from build123d import *

# Parameters (mm, degrees)
SKETCH002_R            = 1.6
PAD_DEPTH              = 2
CHAMFER_SIZE           = 1.65
CHAMFER003_SIZE        = 1.65
SKETCH005_W            = 15.232
SKETCH005_H            = 21.56
SKETCH005_W_2          = 2.5
SKETCH005_H_2          = 2.6
PAD003_DEPTH           = 2
SKETCH_R               = 3.8
SKETCH_R_2             = 1.6
PAD004_DEPTH           = 4.3
SKETCH001_W            = 15.232
SKETCH001_H            = 20
SKETCH001_R            = 1.1
PAD001_DEPTH           = 2
CHAMFER002_SIZE        = 1.2
FUSION_PLACEMENT_ANGLE = 180


with BuildPart() as chamfer003:
    # Sketch002 → Pad (new body)
    with BuildSketch(Plane.XY):
        with BuildLine():
            ThreePointArc((15.232, 41.56), (7.616, 49.176), (0, 41.56))
            Line((0, 41.56), (15.232, 41.56))
        make_face()
        with Locations((7.616, 45.28)):
            Circle(SKETCH002_R, mode=Mode.SUBTRACT)
        with BuildLine():
            ThreePointArc((0, -20), (7.616, -27.616), (15.232, -20))
            Line((0, -20), (15.232, -20))
        make_face()
        with Locations((7.616, -23.72)):
            Circle(SKETCH002_R, mode=Mode.SUBTRACT)
    extrude(amount=PAD_DEPTH)

    # Chamfer
    chamfer_edges = [chamfer003.edges().sort_by_distance(p)[0] for p in [
        (6.016, 45.28, 0),
    ]]
    chamfer(chamfer_edges, length=CHAMFER_SIZE)

    # Chamfer003
    chamfer003_edges = [chamfer003.edges().sort_by_distance(p)[0] for p in [
        (6.016, -23.72, 0),
    ]]
    chamfer(chamfer003_edges, length=CHAMFER003_SIZE)


with BuildPart() as pad003:
    # Sketch005 → Pad003 (new body)
    with BuildSketch(Plane.XY):
        with Locations((7.616, 10.78)):
            Rectangle(SKETCH005_W, SKETCH005_H)
        with Locations((2.3099, 10.78)):
            Rectangle(SKETCH005_W_2, SKETCH005_H_2, mode=Mode.SUBTRACT)
        with Locations((2.3099, 14.03)):
            Rectangle(SKETCH005_W_2, SKETCH005_H_2, mode=Mode.SUBTRACT)
        with Locations((2.3099, 7.53)):
            Rectangle(SKETCH005_W_2, SKETCH005_H_2, mode=Mode.SUBTRACT)
        with Locations((5.2399, 14.03)):
            Rectangle(SKETCH005_W_2, SKETCH005_H_2, mode=Mode.SUBTRACT)
        with Locations((5.2399, 10.78)):
            Rectangle(SKETCH005_W_2, SKETCH005_H_2, mode=Mode.SUBTRACT)
        with Locations((5.2399, 7.53)):
            Rectangle(SKETCH005_W_2, SKETCH005_H_2, mode=Mode.SUBTRACT)
        with Locations((10, 14.03)):
            Rectangle(SKETCH005_W_2, SKETCH005_H_2, mode=Mode.SUBTRACT)
        with Locations((12.93, 14.03)):
            Rectangle(SKETCH005_W_2, SKETCH005_H_2, mode=Mode.SUBTRACT)
        with Locations((10, 10.78)):
            Rectangle(SKETCH005_W_2, SKETCH005_H_2, mode=Mode.SUBTRACT)
        with Locations((12.93, 10.78)):
            Rectangle(SKETCH005_W_2, SKETCH005_H_2, mode=Mode.SUBTRACT)
        with Locations((10, 7.53)):
            Rectangle(SKETCH005_W_2, SKETCH005_H_2, mode=Mode.SUBTRACT)
        with Locations((12.93, 7.53)):
            Rectangle(SKETCH005_W_2, SKETCH005_H_2, mode=Mode.SUBTRACT)
    extrude(amount=PAD003_DEPTH)


with BuildPart() as pad004:
    # Sketch → Pad004 (new body)
    with BuildSketch(Plane.XY.offset(2)):
        with Locations((7.616, 45.28)):
            Circle(SKETCH_R)
        with Locations((7.616, 45.28)):
            Circle(SKETCH_R_2, mode=Mode.SUBTRACT)
        with Locations((7.616, -23.72)):
            Circle(SKETCH_R)
        with Locations((7.616, -23.72)):
            Circle(SKETCH_R_2, mode=Mode.SUBTRACT)
    extrude(amount=PAD004_DEPTH)


with BuildPart() as fusion:
    # Sketch001 → Pad001 (new body)
    with BuildSketch(Plane.XY):
        with Locations((7.616, -10)):
            Rectangle(SKETCH001_W, SKETCH001_H)
        with Locations((3.8995, -16.9419)):
            Circle(SKETCH001_R, mode=Mode.SUBTRACT)
        with Locations((11.3325, -16.9419)):
            Circle(SKETCH001_R, mode=Mode.SUBTRACT)
        with Locations((7.616, 31.56)):
            Rectangle(SKETCH001_W, SKETCH001_H)
        with Locations((3.8995, 38.5019)):
            Circle(SKETCH001_R, mode=Mode.SUBTRACT)
        with Locations((11.3325, 38.5019)):
            Circle(SKETCH001_R, mode=Mode.SUBTRACT)
    extrude(amount=PAD001_DEPTH)

    # Chamfer002
    chamfer002_edges = [fusion.edges().sort_by_distance(p)[0] for p in [
        (10.2325, -16.9419, 0),
        (2.7995, -16.9419, 0),
        (10.2325, 38.5019, 0),
        (2.7995, 38.5019, 0),
    ]]
    chamfer(chamfer002_edges, length=CHAMFER002_SIZE)

    # Fusion: union Chamfer003, Pad003, Pad004
    add(chamfer003.part)
    add(pad003.part)
    add(pad004.part)


with BuildPart() as fusion_1:
    # Fusion placement: moved
    add(fusion.part.moved(Location((0, 0, 40))).rotate(Axis((0, 0, 40), (1, 0, 0)), FUSION_PLACEMENT_ANGLE))


solid = fusion_1.part
Input: part model. Units: mm. Frame: model coordinates. A direction names the side the tool comes from. Coordinates: 2 decimals unless noted, no trailing zeros. Loops run counter-clockwise (first coordinate to the right, second up) from the corner with the lowest first, then second, coordinate; pieces in that order, holes last.
(1) Section B-B on z = 37. Return the cut outline in (x, y), then the cut area to 3 significant figures.
(2) Material intervals for probe 1 along X at (y, z) = (-14, 38.75); probe 2 along Y at (x, z) = (12.75, 39.5); probe 3 along Y at (x, z) = (1.75, 39.75), sorted ascending.
(3) Set-up query: faces 1 (the face through (9, -44, 33.7)), 2 (the face through (14.18, -11, 39)). Return all of +Z, -Z, +X, -X, +Y, -Y with unobstructed straight access to the full face (end or side cutting, diameter ignored); none if empty.
(4) Pull-direction query (Y, two-part tool) for faces 3 (the face through (3.56, -11, 39)), 4 (the face through (9, 25, 33.7)); classes: released by +Y, released by -Y, zero draft, split by the parting line, or undercut.
(5) Section D-D on y = -20.5. Return the cut outline in (x, z).
(6) Section C-C on y = -45.28. Return the cut outline in (x, z).
(7) First-contact query: pin 1 Ø1.6 at (x, z) = (10.5, 38.5) entering from -Y; pin 2 Ø1.6 at (x, z) = (2, 39.5) entering from -Y; pin 3 Ø1 at (x, z) = (5, 39) entering from +Y; pin 4 Ø0.6 at (y, z) = (-10.5, 38.5) entering from -X. Flat tips, straight axial feed; report the tip coordinate or a pass-through.
(8) Section A-A on y = -10.5. Return the cut outline in (x, z), then the cut area to 3 significant figures.
Data:
1. outline: circle Ø7.6 at (7.62, -45.28); circle Ø7.6 at (7.62, 23.72); hole circle Ø3.2 at (7.62, -45.28); hole circle Ø3.2 at (7.62, 23.72)
1. area: 74.6 mm2
2. probe 1: x = 0 to 1.06, 3.56 to 3.99, 6.49 to 8.75, 11.25 to 11.68, 14.18 to 15.23
2. probe 2: y = -47.19 to -39.61, -37.39 to -15.33, -12.73 to -12.08, -9.48 to -8.83, -6.23 to 15.83, 18.05 to 25.63
2. probe 3: y = -46.42 to -15.33, -12.73 to -12.08, -9.48 to -8.83, -6.23 to 24.86
3. face 1: -Z, +X, -X, +Y, -Y
3. face 2: +Z, -Z
4. face 3: undercut
4. face 4: zero draft
5. outline: (0, 38) - (15.23, 38) - (15.23, 40) - (0, 40) - close
6. outline: (0.97, 38) - (3.82, 38) - (3.82, 33.7) - (6.02, 33.7) - (6.02, 38.35) - (4.37, 40) - (0.97, 40) - close; (9.22, 33.7) - (11.42, 33.7) - (11.42, 38) - (14.26, 38) - (14.26, 40) - (10.87, 40) - (9.22, 38.35) - close
7. pin 1: stops at y = -48.89
7. pin 2: stops at y = -47.46
7. pin 3: stops at y = 27.32
7. pin 4: stops at x = 0
8. outline: (0, 38) - (1.06, 38) - (1.06, 40) - (0, 40) - close; (3.56, 38) - (3.99, 38) - (3.99, 40) - (3.56, 40) - close; (6.49, 38) - (8.75, 38) - (8.75, 40) - (6.49, 40) - close; (11.25, 38) - (11.68, 38) - (11.68, 40) - (11.25, 40) - close; (14.18, 38) - (15.23, 38) - (15.23, 40) - (14.18, 40) - close
8. area: 10.5 mm2
